Model file for the job. Use its own axes, mm. Give positions to 0.01 mm unless a question says otherwise; leave off trailing zeros. Write each loop counter-clockwise with the first axis right and the second up, starting at its lowest first coordinate (ties: lowest second). Pieces come first, ordered by that corner, then holes.
```python
from build123d import *

# Parameters (mm, degrees)
SKETCH1_W                                           = 32.5
SKETCH1_H                                           = 30
BOSS_EXTRUDE1_DEPTH                                 = 5
CSK_FOR_M3_COUNTERSUNK_FLAT_HEAD_SCREW1_D           = 3.3
CSK_FOR_M3_COUNTERSUNK_FLAT_HEAD_SCREW1_CSINK_D     = 5.8
CSK_FOR_M3_COUNTERSUNK_FLAT_HEAD_SCREW1_CSINK_ANGLE = 90


with BuildPart() as part:
    # Sketch1 → Boss-Extrude1 (new body)
    with BuildSketch(Plane(origin=(0, 0, 0), x_dir=(1, 0, 0), z_dir=(0, 1, 0))):
        Rectangle(SKETCH1_W, SKETCH1_H)
    extrude(amount=BOSS_EXTRUDE1_DEPTH)

    # Sketch3 → CSK for M6 Hex Socket Countersunk Cap Screw1 (revolve, cut)
    with BuildSketch(Plane(origin=(0, 0, 0), x_dir=(0, 0, -1), z_dir=(1, 0, 0))):
        Polygon((0, 0), (0, 5), (3.15, 5), (3.15, 3.1), (6.25, 0), align=None)
    revolve(axis=Axis((0, -6.35, 0), (0, 1, 0)), mode=Mode.SUBTRACT)

    # CSK for M3 Countersunk Flat Head Screw1 (through all)
    with Locations(Plane(origin=(0, 5, 0), x_dir=(1, 0, 0), z_dir=(0, 1, 0))):
        with Locations((0, 0), (10, -10), (-10, 10), (-10, -10), (10, 10)):
            CounterSinkHole(CSK_FOR_M3_COUNTERSUNK_FLAT_HEAD_SCREW1_D / 2, CSK_FOR_M3_COUNTERSUNK_FLAT_HEAD_SCREW1_CSINK_D / 2, counter_sink_angle=CSK_FOR_M3_COUNTERSUNK_FLAT_HEAD_SCREW1_CSINK_ANGLE)


solid = part.part
```
1. Probe probe 1 along Z at (x, y) = (10, 1); probe 2 along X at (y, z) = (2.7, 10); probe 3 along Z at (x, y) = (10.5, 4.2). List the from-to ranges inside material, lowest first.
Calculated:
probe 1: z = -15 to -11.65, -8.35 to 8.35, 11.65 to 15
probe 2: x = -16.25 to -11.65, -8.35 to 8.35, 11.65 to 16.25
probe 3: z = -15 to -12.04, -7.96 to 7.96, 12.04 to 15
2. Slice it at A-A, the plane z = -10. Write the cut outline in (x, y), and give its area (3 significant figures).
Calculated:
outline: (-16.25, 0) - (-11.65, 0) - (-11.65, 3.75) - (-12.9, 5) - (-16.25, 5) - close; (-8.35, 0) - (8.35, 0) - (8.35, 3.75) - (7.1, 5) - (-7.1, 5) - (-8.35, 3.75) - close; (11.65, 0) - (16.25, 0) - (16.25, 5) - (12.9, 5) - (11.65, 3.75) - close
area: 126 mm2
3. Slice it at C-C, the plane x = 10. Write the cut outline in (y, z), and give its area (3 significant figures).
Calculated:
outline: (0, -15) - (5, -15) - (5, -12.9) - (3.75, -11.65) - (0, -11.65) - close; (0, -8.35) - (3.75, -8.35) - (5, -7.1) - (5, 7.1) - (3.75, 8.35) - (0, 8.35) - close; (0, 11.65) - (3.75, 11.65) - (5, 12.9) - (5, 15) - (0, 15) - close
area: 114 mm2
4. Pin check, flat tip, straight feed: P1, Ø4.5, axis at x = -10, z = -10, coming from the +Y side. Stop position of the tip, or through.
Calculated:
P1: stops at y = 4.35
5. Pull direction Z, two halves, no side cores. Call faces 1 (the flat face through (0, 2, 15)), 2 (the flat face through (-16.25, 2, 0)), 3 (the conical face through (-1, 2.9, -3.2)), 4 (the flat face through (0, 2, -15)): +Z half, -Z half, draft (parallel to the pull), parting line (faces both ways), or undercut.
Calculated:
face 1: +Z half
face 2: draft
face 3: undercut
face 4: -Z half
6. Slice it at B-B, the plane y = 4.55. Write the cut outline in (x, z), and give its area (3 significant figures).
Calculated:
outline: (-16.25, -15) - (16.25, -15) - (16.25, 15) - (-16.25, 15) - close; hole circle Ø4.9 at (-10, -10); hole circle Ø4.9 at (-10, 10); hole circle Ø6.3 at (0, 0); hole circle Ø4.9 at (10, -10); hole circle Ø4.9 at (10, 10)
area: 868 mm2
7. Slice it at D-D, the plane z = 0. Write the cut outline in (x, y), and give its area (3 significant figures).
Calculated:
outline: (-16.25, 0) - (-6.25, 0) - (-3.15, 3.1) - (-3.15, 5) - (-16.25, 5) - close; (3.15, 3.1) - (6.25, 0) - (16.25, 0) - (16.25, 5) - (3.15, 5) - close
area: 121 mm2
